Source: CAD feature listing. Evaluate the final solid. Frame: model axes, mm. Face numbers are marked on the shaded views. Round coordinates to 2 decimals unless told otherwise and drop trailing zeros. Order: outer loops, then holes, each group sorted by start corner. A loop starts at its lowest first (then second) coordinate and runs counter-clockwise, first axis right, second up. Notation, with made-up numbers: M 57.25,35 L 92.25,35 A31 ccw 92.25,62 Z; hole C 50,19.25 d3. An arc over 180 degrees is marked long. Answer as CSV lines item,"result". Start each with the question number.
Item 1: Line query: line 1 (Z direction, x = -10, y = 2.6); line 2 (X direction, y = 1, z = 6.5); line 3 (X direction, y = 1.7, z = 0.5). Output: solid intervals per line, ascending. Write a range as [from, to].
Item 2: Section query C-C on y = 1.55. Return the cut outline in (x, z).
Item 3: Section query D-D on x = -1. Return the cut outline in (y, z).
Item 4: Section query A-A on z = 17.5. Return the cut outline in (x, y).
Item 5: Pull-direction query (Y, two-part tool) for the marked faces 1 and 2; classes: +Y half, -Y half, draft (parallel to the pull), parting line (faces both ways), or undercut.
Item 6: Section query B-B on x = 5. Return the cut outline in (y, z).
Item 7: First-contact query: P1, Ø1.4, axis at x = -30, y = 2, coming from the +Z side; P2, Ø0.9, axis at x = 10, y = 1, coming from the -Z side; P3, Ø0.9, axis at x = -29.5, y = 1, coming from the -Z side. Flat tips, straight axial feed; report the tip coordinate or a pass-through.
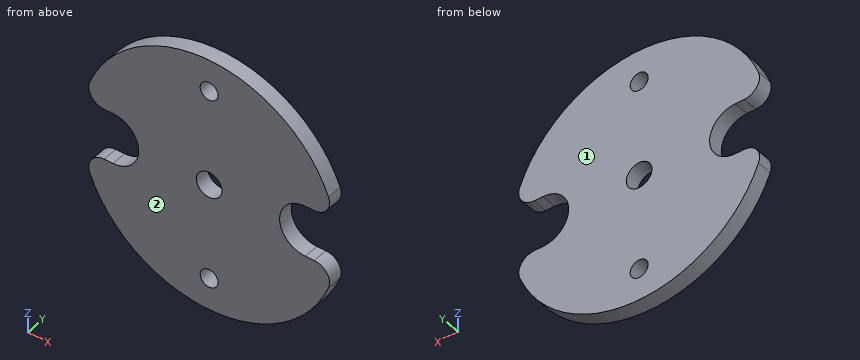
from build123d import *

# Parameters (mm, degrees)
SKETCH1_R           = 1.778
SKETCH1_R_2         = 2.54
BOSS_EXTRUDE1_DEPTH = 3.048


with BuildPart() as part:
    # Sketch1 → Boss-Extrude1 (new body)
    with BuildSketch(Plane(origin=(0, 0, 0), x_dir=(1, 0, 0), z_dir=(0, 1, 0))):
        with BuildLine():
            Line((-28.837830229, 5.581683581), (-30.609634186, 5.581683581))
            ThreePointArc((-30.609634186, 5.581683581), (-33.126437353, 6.910379705), (-33.448971089, 9.738047217))
            ThreePointArc((-33.448971089, 9.738047217), (-9.787830229, 25.901683581), (13.87331063, 9.738047217))
            ThreePointArc((13.87331063, 9.738047217), (13.550776894, 6.910379705), (11.033973727, 5.581683581))
            Line((11.033973727, 5.581683581), (9.262169771, 5.581683581))
            ThreePointArc((9.262169771, 5.581683581), (4.182169771, 0.501683581), (9.262169771, -4.578316419))
            Line((9.262169771, -4.578316419), (11.033973727, -4.578316419))
            ThreePointArc((11.033973727, -4.578316419), (13.550776894, -5.907012543), (13.87331063, -8.734680055))
            ThreePointArc((13.87331063, -8.734680055), (-9.787830229, -24.898316419), (-33.448971089, -8.734680055))
            ThreePointArc((-33.448971089, -8.734680055), (-33.126437353, -5.907012543), (-30.609634186, -4.578316419))
            Line((-30.609634186, -4.578316419), (-28.837830229, -4.578316419))
            ThreePointArc((-28.837830229, -4.578316419), (-23.757830229, 0.501683581), (-28.837830229, 5.581683581))
        make_face()
        with Locations(Location((-9.787830229, 19.551683581, 0), (0, 0, 90))):
            Circle(SKETCH1_R, mode=Mode.SUBTRACT)
        with Locations(Location((-9.787830229, -18.548316419, 0), (0, 0, 90))):
            Circle(SKETCH1_R, mode=Mode.SUBTRACT)
        with Locations(Location((-9.787830229, 0.501683581, 0), (0, 0, 90))):
            Circle(SKETCH1_R_2, mode=Mode.SUBTRACT)
    extrude(amount=BOSS_EXTRUDE1_DEPTH)


solid = part.part
Results:
1,line 1,"[-25.9, -21.32], [-17.79, -3.03], [2.03, 16.78], [20.31, 24.9]"
1,line 2,"[-33.44, 13.87]"
1,line 3,"[-23.86, -12.12], [-7.45, 4.28]"
2,outline,"M -33.45,-9.74 A25.4 ccw 13.87,-9.74 A3.05 ccw 11.03,-5.58 L 9.26,-5.58 A5.08 cw 9.26,4.58 L 11.03,4.58 A3.05 ccw 13.87,8.73 A25.4 ccw -33.45,8.73 A3.05 ccw -30.61,4.58 L -28.84,4.58 A5.08 cw -28.84,-5.58 L -30.61,-5.58 A3.05 ccw Z; hole C -9.79,-0.5 d5.08; hole C -9.79,-19.55 d3.56; hole C -9.79,18.55 d3.56"
3,outline,"M 0,-24.33 L 3.05,-24.33 L 3.05,23.33 L 0,23.33 Z"
4,outline,"M -27.71,0 L -11.22,0 L -11.22,3.05 L -27.71,3.05 Z; M -8.35,0 L 8.13,0 L 8.13,3.05 L -8.35,3.05 Z"
5,face 1,"+Y half"
5,face 2,"-Y half"
6,outline,"M 0,-21.15 L 3.05,-21.15 L 3.05,-3.27 L 0,-3.27 Z; M 0,2.26 L 3.05,2.26 L 3.05,20.15 L 0,20.15 Z"
7,P1,"z = 15.76"
7,P2,"z = -16.97"
7,P3,"z = -17.06"
